Here's how the part is built. I have some questions about the finished solid (model axes, mm). A direction names the side the tool comes from. Round coordinates to 2 decimals unless told otherwise and drop trailing zeros. Order: outer loops, then holes, each group sorted by start corner. A loop starts at its lowest first (then second) coordinate and runs counter-clockwise, first axis right, second up. Notation, with made-up numbers: M 19.5,22 L 70.5,22 A14 ccw 70.5,32 Z; hole C 80,28.5 d2. An arc over 180 degrees is marked long. Use one line per item in the form item = value. Start each with the question number.
Autodesk Inventor part; units mm, degrees
ref_plane "YZ Plane" through (0, 0, 0) normal (1, 0, 0) x (0, 1, 0)
ref_plane "XZ Plane" through (0, 0, 0) normal (0, 1, 0) x (-1, 0, 0)
ref_plane "XY Plane" through (0, 0, 0) normal (0, 0, 1) x (1, 0, 0)
sketch "Sketch1" plane through (0, 0, 0) normal (0, 1, 0) x (-1, 0, 0)
  line L0 (-8.5, -155) -> (8.5, -155)
  line L1 (8.5, -155) -> (8.5, 155)
  line L2 (8.5, 155) -> (-8.5, 155)
  line L3 (-8.5, 155) -> (-8.5, -155)
  line L4 (-8.5, -155) -> (8.5, 155) construction
  line L5 (8.5, -155) -> (-8.5, 155) construction
  point P0 (0, 0)
  dimension "d0" = 310
  dimension "d1" = 17
extrude "Extrusion1" add sketch "Sketch1" along normal blind 4.4
chamfer "Chamfer1" distance 5 distance2 2 1 edges at (8.5, 4.4, 0) measured on face at (2.8333, 4.4, 51.6667)
chamfer "Chamfer2" distance 5 distance2 2 1 edges at (-8.5, 4.4, 0) measured on face at (-4.5, 4.4, 51.6667)
sketch "Sketch2" plane through (0, 0, 0) normal (0, -1, 0) x (1, 0, 0)
  line L0 (-8.5, -155) -> (-8.5, 155)
  line L1 (8.5, -155) -> (-8.5, -155)
  line L2 (8.5, 155) -> (8.5, -155)
  line L3 (-8.5, 155) -> (8.5, 155)
  circle A0 centre (-5, -158.5) radius 1.75
  circle A1 centre (5, 158.5) radius 1.75
  line L4 (-8.5, 155) -> (8.5, 155)
  line L5 (8.5, 155) -> (8.5, 162)
  line L6 (8.5, 162) -> (-0.5, 162)
  line L7 (-0.5, 162) -> (-0.5, 155)
  line L8 (-8.5, -155) -> (-8.5, 155)
  line L9 (-8.5, -155) -> (-8.5, -162)
  line L10 (-8.5, -162) -> (0.5, -162)
  line L11 (0.5, -162) -> (0.5, -155)
  line L12 (8.5, -155) -> (-8.5, -155)
  point P0 (0, 0)
  dimension "d10" = 3.5
  dimension "d11" = 3.5
  dimension "d12" = 3.5
  dimension "d13" = 3.5
  dimension "d14" = 3.5
  dimension "d15" = 9
  dimension "d16" = 7
extrude "Extrusion2" add sketch "Sketch2" against normal blind 1 contours L1 L11 L10 L9 | L7 L6 L5 L3
sketch "Sketch3" plane through (0, 0, 0) normal (0, -1, 0) x (1, 0, 0)
  circle A0 centre (5, 158.5) radius 1.75
  circle A1 centre (-5, -158.5) radius 1.75
  line L0 (-8.5, -162) -> (-8.5, 155)
  line L1 (-8.5, -162) -> (0.5, -162)
  line L2 (0.5, -162) -> (0.5, -155)
  line L3 (8.5, -155) -> (0.5, -155)
  line L4 (8.5, -155) -> (8.5, 162)
  line L5 (8.5, 162) -> (-0.5, 162)
  line L6 (-0.5, 162) -> (-0.5, 155)
  line L7 (-8.5, 155) -> (-0.5, 155)
  line L8 (5.5, -152) -> (-5.5, -152)
  line L9 (-5.5, -152) -> (-5.5, 152)
  line L10 (-5.5, 152) -> (5.5, 152)
  line L11 (5.5, 152) -> (5.5, -152)
  line L12 (8.5, -155) -> (0.5, -155)
  point P0 (0, 0)
  point P1 (4.5, -155)
  dimension "d19" = 3
  dimension "d20" = 3
  dimension "d21" = 3
  dimension "d22" = 3
extrude "Extrusion3" cut sketch "Sketch3" against normal blind 1 contours L8 L9 L10 L11
equation "\"d11\" = d10"
equation "\"d13\" = d10"
equation "\"d14\" = d10"
equation "\"d16\" = 2 * d14"
equation "\"d20\" = d19"
equation "\"d21\" = d19"
properties part number "ZLF Alumiline 310" material "Aluminum 6061"
1) On a 3-axis mill with a long thin cutter (end or side, diameter ignored), from which of +Z, -Z, +X, -X, +Y, -Y can I reach the whole of each face in a straight line? I mean faces 1 (the flat face through (3, 1, 159)), 2 (the flat face through (6, 0, 2)). Say none if no direction works.
2) If I drill on line 1 (Z direction, x = 5, y = 0.55); line 2 (Z direction, x = -5, y = 0.8); line 3 (X direction, y = 0.5, z = -158.5), over which ranges is the centre line in solid material (lowest first)?
3) If we mould it in two halves opening along X, with no side actions, what happens to faces 3 (the flat face through (-3, 1, -158)), 4 (the flat face through (-6, 3.4, -2.2)), 5 (the flat face through (6, 3.4, 2.2)), 6 (the flat face through (0, 1, 2))? For each: +X half, -X half, draft (parallel to the pull), parting line (faces both ways), or undercut.
4) Will these pins go through, and if not, where does the flat tip stop? pin 1 Ø5 at (x, z) = (-6.5, -108) entering from +Y; pin 2 Ø0.8 at (x, y) = (2.5, 0.5) entering from -Z; pin 3 Ø3 at (x, z) = (-2.5, 108) entering from -Y.
5) If we section it at A-A on z = 32.5: Write out the boundary of the cut face in (x, y).
Completed:
q1.face_1 = +Z, +X, -X, +Y
q1.face_2 = +Z, -Z, +X, -X, -Y
q2.line_1 = -155 to -152, 152 to 156.75, 160.25 to 162
q2.line_2 = -162 to -160.25, -156.75 to -152, 152 to 155
q2.line_3 = -8.5 to -6.75, -3.25 to 0.5
q3.face_3 = draft
q3.face_4 = -X half
q3.face_5 = +X half
q3.face_6 = undercut
q4.pin_1 = 4.2
q4.pin_2 = -155
q4.pin_3 = 1
q5.outline = M -8.5,0 L -5.5,0 L -5.5,1 L 5.5,1 L 5.5,0 L 8.5,0 L 8.5,2.4 L 3.5,4.4 L -3.5,4.4 L -8.5,2.4 Z
